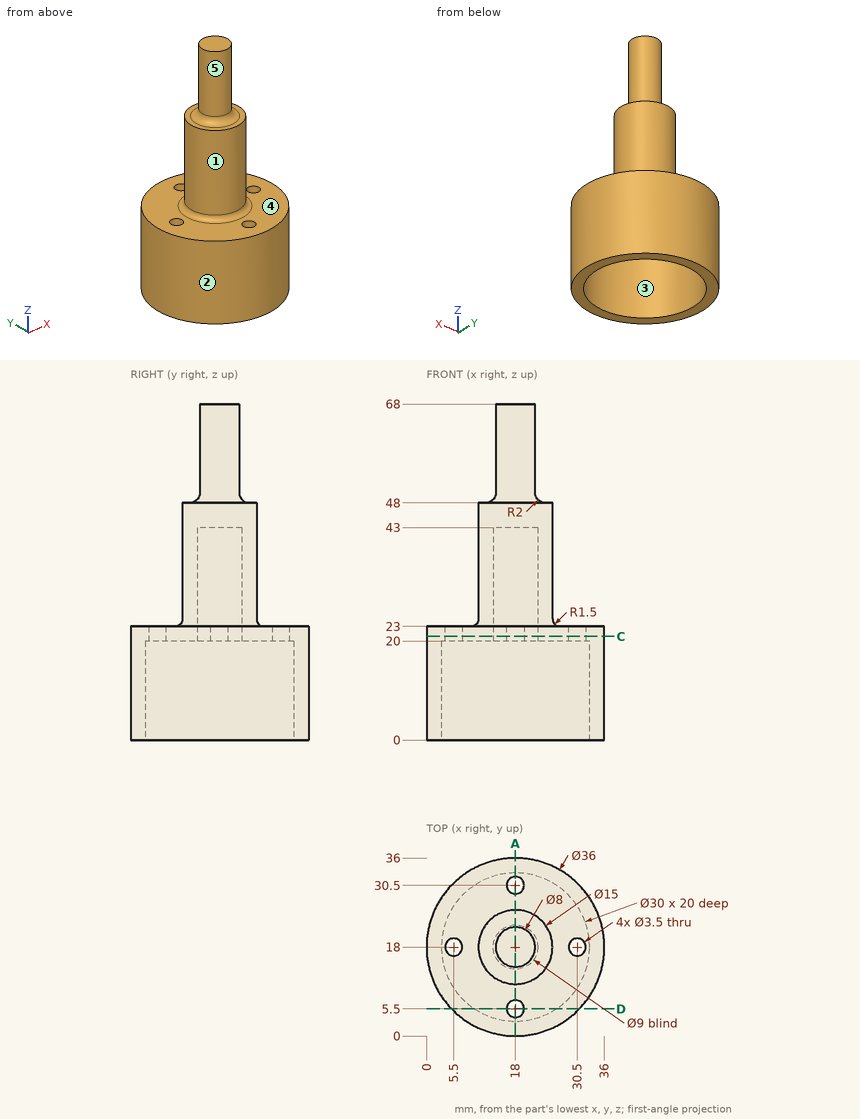
Geometry: see drawing. Coordinates: mm, zero at the bounding-box minimum. A direction names the side the tool comes from. Give positions to 0.01 mm unless a question says otherwise; leave off trailing zeros. Order: outer loops, then holes, each group sorted by start corner. A loop starts at its lowest first (then second) coordinate and runs counter-clockwise, first axis right, second up. Notation, with made-up numbers: (41, 14.5) -> (81, 14.5) arc R29 cw to (81, 40.5) -> close; hole circle Ø1 at (56.5, 54.25). An arc over 180 degrees is marked (long way). Write item = value, one per line.
Q1. Set-up query: the marked faces 1 and 2. Return all of +Z, -Z, +X, -X, +Y, -Y with unobstructed straight access to the full face (end or side cutting, diameter ignored); none if empty.
Data:
face_1 = +Z
face_2 = +Z, -Z
Q2. Material intervals for line 1 (Y direction, x = 18, z = 22.15); line 2 (Y direction, x = 18, z = 31); line 3 (X direction, y = 31.5, z = 10.5), sorted ascending. Write a range as from..to.
Data:
line_1 = 0..3.75, 7.25..13.5, 22.5..28.75, 32.25..36
line_2 = 10.5..13.5, 22.5..25.5
line_3 = 6.09..11.46, 24.54..29.91
Q3. Pin query (flat end, axial travel): pin 1 (5.5 mm diameter, centred on x = 5.5, y = 18, fed in from -Z); pin 2 (5.5 mm diameter, centred on x = 30.5, y = 18, fed in from +Z); pin 3 (8 mm diameter, centred on x = 16.5, y = 28, fed in from -Z); pin 4 (11 mm diameter, centred on x = 27, y = 25, fed in from +Z). Return the tip coordinate at first contact, or that it passes through.
Data:
pin_1 = 0
pin_2 = 23
pin_3 = 20
pin_4 = 48
Q4. Pull-direction query (Y, two-part tool) for the marked faces 3, 4 and 5; classes: released by +Y, released by -Y, zero draft, split by the parting line, or undercut.
Data:
face_3 = undercut
face_4 = zero draft
face_5 = split by the parting line
Q5. Cut plane D-D, the plane y = 5.5. Output: boundary loops of the cut face in (x, z), and give its area (3 significant figures).
Data:
outline = (5.05, 0) -> (9.71, 0) -> (9.71, 20) -> (16.25, 20) -> (16.25, 23) -> (5.05, 23) -> close; (19.75, 20) -> (26.29, 20) -> (26.29, 0) -> (30.95, 0) -> (30.95, 23) -> (19.75, 23) -> close
area = 254 mm^2
Q6. Cut plane C-C, the plane z = 21. Output: boundary loops of the cut face in (x, y), and give its area (3 significant figures).
Data:
outline = circle Ø36 at (18, 18); hole circle Ø3.5 at (5.5, 18); hole circle Ø9 at (18, 18); hole circle Ø3.5 at (18, 5.5); hole circle Ø3.5 at (18, 30.5); hole circle Ø3.5 at (30.5, 18)
area = 916 mm^2
Q7. Cut plane A-A, the plane x = 18. State how many separate pieces and enclosed holes the cut face has, and give its area (3 significant figures).
Data:
separate_pieces = 3
enclosed_holes = 0
area = 538 mm^2
